The listing builds one solid part. Answer for the finished solid, in the listing's coordinates (mm). A direction names the side the tool comes from. Give positions to 0.01 mm unless a question says otherwise; leave off trailing zeros. Loops run counter-clockwise (first coordinate to the right, second up) from the corner with the lowest first, then second, coordinate; pieces in that order, holes last. Notation, with made-up numbers: (75.5, 81.25) - (112.5, 81.25) arc R10 cw to (112.5, 93.25) - close; hole circle Ø8 at (45.5, 53.25). An arc over 180 degrees is marked (long way). Write each question's results on one line, items separated by ' | '.
from build123d import *

# Parameters (mm, degrees)
F1_DEPTH   = 1.27
F2_SIZE2   = 0.635
F2_SIZE    = 5.08
F2_2_SIZE2 = 0.63499
F2_2_SIZE  = 5.07999


# Not quite as in the source:
# - a fillet or chamfer is up to 0.001 mm smaller than in the source, because OpenCascade refuses the exact size


with BuildPart() as f1:
    # F0 (on Top) → F1 (new body)
    with BuildSketch(Plane.XY):
        with BuildLine():
            Line((-36.8330654015, 25.4), (-36.8330654015, 0))
            Line((-36.8330654015, 0), (-31.7530654015, 0))
            Line((-31.7530654015, 0), (-31.7530654015, 25.4))
            Line((-31.7530654015, 25.4), (-31.7530654015, 38.1))
            Line((-31.7530654015, 38.1), (-34.0151443949, 52.5287568289))
            ThreePointArc((-34.0151443949, 52.5287568289), (-30.3739911163, 64.9655644869), (-36.8330654015, 76.2))
            Line((-36.8330654015, 76.2), (-36.8330654015, 25.4))
        make_face()
    extrude(amount=F1_DEPTH)

    # F2
    f2_edges = [f1.edges().sort_by_distance(p)[0] for p in [
        (-30.373991, 64.965564, 1.27),
    ]]
    f2_side = f1.faces().sort_by_distance((-34.308504, 37.141649, 1.27))[0]
    chamfer(f2_edges, length=F2_SIZE, length2=F2_SIZE2, reference=f2_side)

    # F2#2 (size 5.08 and 0.635 in the source; OpenCascade refuses exactly that, so slightly less here)
    f2_2_edges = [f1.edges().sort_by_distance(p)[0] for p in [
        (-30.373991, 64.965564, 0),
    ]]
    f2_2_side = f1.faces().sort_by_distance((-34.308504, 37.141649, 0))[0]
    chamfer(f2_2_edges, length=F2_2_SIZE, length2=F2_2_SIZE2, reference=f2_2_side)


solid = f1.part
Item 1: For faces 4 (the face through (-34, 27, 1.27)), 5 (the face through (-31.753, 19, 1)), determine the directions among +Z, -Z, +X, -X, +Y, -Y from which every point of the face is accessible in a straight line to the end or side of a thin tool.
Values found:
face 4: +Z, +X, -X, +Y, -Y | face 5: +Z, -Z, +X, -Y
Item 2: A cutting plane is placed at C-C, the plane y = 39. Determine the outline of the cut face in (x, z), plus the area to 3 significant figures.
Values found:
outline: (-36.83, 0) - (-31.89, 0) - (-31.89, 1.27) - (-36.83, 1.27) - close | area: 6.27 mm²
Item 3: Find the intervals of material crossed by line 1 along X through (y, z) = (12.5, 0.95); line 2 along X through (y, z) = (42.5, 0.2), in increasing order. Write a range as [from, to].
Values found:
line 1: x = [-36.83, -31.75] | line 2: x = [-36.83, -32.44]
Item 4: A cutting plane is placed at A-A, the plane z = 0.2. Determine the outline of the cut face in (x, y), plus the area to 3 significant figures.
Values found:
outline: (-36.83, 0) - (-31.75, 0) - (-31.75, 38.1) - (-34.84, 57.78) arc R13.03 ccw to (-36.83, 71.44) - close | area: 295 mm²
Item 5: For a pull along Y with two mould halves and no side action, classify faces 1 (the face through (-34, 0, 1)), 2 (the face through (-33.4, 64.45, 1.02)), 3 (the face through (-36.833, 39, 1)) as released by +Y, released by -Y, zero draft, split by the parting line, or undercut.
Values found:
face 1: released by -Y | face 2: undercut | face 3: zero draft
Item 6: A cutting plane is placed at B-B, the plane y = 28.5. Determine the outline of the cut face in (x, z).
Values found:
outline: (-36.83, 0) - (-31.75, 0) - (-31.75, 1.27) - (-36.83, 1.27) - close
Item 7: A flat-ended cylindrical pin translates along its axis: P1, Ø1, axis at x = -34.5, y = 60, coming from the +Z side. Find the tip coordinate at first contact, or state that the pin passes through.
Values found:
P1: stops at z = 1.18
